```python
from build123d import *

# Parameters (mm, degrees)
CROQUIS1_W              = 24
CROQUIS1_H              = 10
CROQUIS1_R              = 1.65
SALIENTE_EXTRUIR1_DEPTH = 10.5


with BuildPart() as part:
    # Croquis1 → Saliente-Extruir1 (new body)
    with BuildSketch(Plane.XY):
        Rectangle(CROQUIS1_W, CROQUIS1_H)
        with Locations(Location((-9, 0, 0), (0, 0, 180))):
            Circle(CROQUIS1_R, mode=Mode.SUBTRACT)
        with Locations(Location((9, 0, 0), (0, 0, 180))):
            Circle(CROQUIS1_R, mode=Mode.SUBTRACT)
    extrude(amount=SALIENTE_EXTRUIR1_DEPTH)

    # Croquis2 → Cortar-Revolución1 (revolve, cut)
    with BuildSketch(Plane(origin=(0, 0, 0), x_dir=(0, 0, -1), z_dir=(1, 0, 0))):
        Polygon((-6.5, 1.9), (-6.5, -1.9), (-4.5, -1.9), (-4.5, -5), (-10.5, -5), (-10.5, 5), (-4.5, 5), (-4.5, 1.9), align=None)
    revolve(axis=Axis((0, 5.062819344, 10.5), (0, 1, 0)), mode=Mode.SUBTRACT)


solid = part.part
```
Input: part model. Units: mm. Frame: model coordinates. A direction names the side the tool comes from. Give positions to 0.01 mm unless a question says otherwise; leave off trailing zeros. Loops run counter-clockwise (first coordinate to the right, second up) from the corner with the lowest first, then second, coordinate; pieces in that order, holes last. Notation, with made-up numbers: M 56.5,65.25 L 69.5,65.25 A19 ccw 69.5,93.25 Z; hole C 19,64 d2. An arc over 180 degrees is marked long. Answer as CSV lines item,"result". Start each with the question number.
1. Line query: L1, parallel to Y at x = -9, z = 3; L2, parallel to X at y = -1, z = 6; L3, parallel to Y at x = -0.75, z = 6.5. Output: solid intervals per line, ascending.
2. Section D-D on x = -5. Return loops of the section in (y, z).
3. Reachability of faces 1 (the face through (0.1, 3.4, 4.5)), 2 (the face through (0, -1.9, 6)), 3 (the face through (0, 0, 0)) from +Z, -Z, +X, -X, +Y, -Y: full face, straight path, thin tool, end or side. Return the list, or none.
4. Pin query (flat end, axial travel): P1, Ø5, axis at x = 0, y = 0, coming from the -Z side. Return the tip coordinate at first contact, or that it passes through.
5. Section A-A on z = 9.25. Return loops of the section in (x, y), plus the area to 3 significant figures.
6. Section B-B on x = -9. Return loops of the section in (y, z).
7. Section C-C on z = 2.25. Return loops of the section in (x, y).
8. Pull-direction query (Y, two-part tool) for faces 4 (the face through (0, -5, 4)), 5 (the face through (10.65, -0.07, 5.18)), 6 (the face through (0, 5, 4)); classes: released by +Y, released by -Y, zero draft, split by the parting line, or undercut.
Computed values:
1,L1,"y = -5 to -1.65, 1.65 to 5"
1,L2,"x = -12 to -10.31, -7.69 to 7.69, 10.31 to 12"
1,L3,"y = -1.9 to 1.9"
2,outline,"M -5,0 L 5,0 L 5,7.18 L 1.9,7.18 L 1.9,10.5 L -1.9,10.5 L -1.9,7.18 L -5,7.18 Z"
3,face 1,"+Z, +Y"
3,face 2,"+Z, -Y"
3,face 3,"-Z, +X, -X, +Y, -Y"
4,P1,"stops at z = 0"
5,outline,"M -12,-5 L -5.87,-5 L -5.87,-1.9 L -3.8,-1.9 L -3.8,1.9 L -5.87,1.9 L -5.87,5 L -12,5 Z; M 3.8,-1.9 L 5.87,-1.9 L 5.87,-5 L 12,-5 L 12,5 L 5.87,5 L 5.87,1.9 L 3.8,1.9 Z; hole C -9,0 d3.3; hole C 9,0 d3.3"
5,area,"121 mm²"
6,outline,"M -5,0 L -1.65,0 L -1.65,10.5 L -5,10.5 Z; M 1.65,0 L 5,0 L 5,10.5 L 1.65,10.5 Z"
7,outline,"M -12,-5 L 12,-5 L 12,5 L -12,5 Z; hole C -9,0 d3.3; hole C 9,0 d3.3"
8,face 4,"released by -Y"
8,face 5,"undercut"
8,face 6,"released by +Y"
